```python
from build123d import *

# Parameters (mm, degrees)
BOSS_EXTRUDE1_DEPTH = 6.35
SKETCH2_R           = 1.27
CUT_EXTRUDE1_DEPTH  = 64.634002359


with BuildPart() as part:
    # Sketch1 → Boss-Extrude1 (new body)
    with BuildSketch(Plane.XY):
        with BuildLine():
            Line((52.3875, -33.02), (52.3875, 33.02))
            ThreePointArc((52.3875, 33.02), (51.643551224, 34.816051224), (49.8475, 35.56))
            Line((49.8475, 35.56), (-49.8475, 35.56))
            ThreePointArc((-49.8475, 35.56), (-51.643551224, 34.816051224), (-52.3875, 33.02))
            Line((-52.3875, 33.02), (-52.3875, -33.02))
            ThreePointArc((-52.3875, -33.02), (-51.643551224, -34.816051224), (-49.8475, -35.56))
            Line((-49.8475, -35.56), (49.8475, -35.56))
            ThreePointArc((49.8475, -35.56), (51.643551224, -34.816051224), (52.3875, -33.02))
        make_face()
        with BuildLine():
            Line((-38.502324621, 28.736218676), (13.971672014, 28.736218676))
            ThreePointArc((13.971672014, 28.736218676), (14.869697627, 28.364244288), (15.241672014, 27.466218676))
            Line((15.241672014, 27.466218676), (15.241672014, 21.89465856))
            ThreePointArc((15.241672014, 21.89465856), (14.869697627, 20.996632948), (13.971672014, 20.62465856))
            Line((13.971672014, 20.62465856), (-38.502324621, 20.62465856))
            ThreePointArc((-38.502324621, 20.62465856), (-39.400350233, 20.996632948), (-39.772324621, 21.89465856))
            Line((-39.772324621, 21.89465856), (-39.772324621, 27.466218676))
            ThreePointArc((-39.772324621, 27.466218676), (-39.400350233, 28.364244288), (-38.502324621, 28.736218676))
        make_face(mode=Mode.SUBTRACT)
        with BuildLine():
            Line((1.27, -9.646243467), (12.539518383, -9.646243467))
            ThreePointArc((12.539518383, -9.646243467), (13.437543995, -10.018217855), (13.809518383, -10.916243467))
            Line((13.809518383, -10.916243467), (13.809518383, -27.94))
            ThreePointArc((13.809518383, -27.94), (13.437543995, -28.838025612), (12.539518383, -29.21))
            Line((12.539518383, -29.21), (1.27, -29.21))
            ThreePointArc((1.27, -29.21), (0.371974388, -28.838025612), (0, -27.94))
            Line((0, -27.94), (0, -10.916243467))
            ThreePointArc((0, -10.916243467), (0.371974388, -10.018217855), (1.27, -9.646243467))
        make_face(mode=Mode.SUBTRACT)
    extrude(amount=BOSS_EXTRUDE1_DEPTH)

    # Sketch2 → Cut-Extrude1 (cut, through all)
    with BuildSketch(Plane.XY.offset(6.35)):
        with Locations((-49.3395, -22.86)):
            Circle(SKETCH2_R)
        with Locations((-49.3395, 22.86)):
            Circle(SKETCH2_R)
        with Locations((49.3395, 22.86)):
            Circle(SKETCH2_R)
        with Locations((49.3395, -22.86)):
            Circle(SKETCH2_R)
    extrude(amount=-CUT_EXTRUDE1_DEPTH, mode=Mode.SUBTRACT)


solid = part.part
```
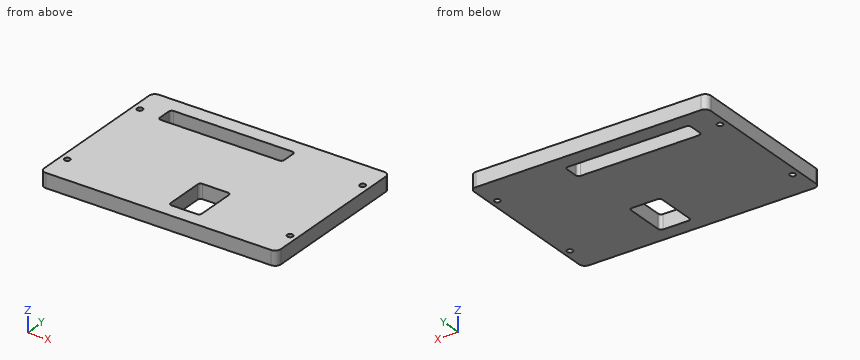
Geometry check sheet. Reference: the model listing, model coordinates, mm. Coordinates: 2 decimals unless noted, no trailing zeros. Order: outer loops, then holes, each group sorted by start corner. A loop starts at its lowest first (then second) coordinate and runs counter-clockwise, first axis right, second up. Notation, with made-up numbers: M 15.5,-10 L 34.5,-10 A17 ccw 34.5,-3 Z; hole C 75.5,-29.75 d2. An arc over 180 degrees is marked long. Answer as a JSON object with one key per item and string values.
Q1. Depth check by flat-ended pin: pin 1 Ø8 at (x, y) = (13.5, 22.5) entering from -Z. Enter the tip coordinate at first touch or a pass-through.
Results are:
{"pin 1": "stops at z = 0"}
Q2. Cross-section at A-A on y = -22.86. Record the cut outline in (x, z).
Results are:
{"outline": "M -52.39,0 L -50.61,0 L -50.61,6.35 L -52.39,6.35 Z; M -48.07,0 L 0,0 L 0,6.35 L -48.07,6.35 Z; M 13.81,0 L 48.07,0 L 48.07,6.35 L 13.81,6.35 Z; M 50.61,0 L 52.39,0 L 52.39,6.35 L 50.61,6.35 Z"}
Q3. Cross-section at B-B on z = 2. Record the cut outline in (x, y).
Results are:
{"outline": "M -52.39,-33.02 A2.54 ccw -49.85,-35.56 L 49.85,-35.56 A2.54 ccw 52.39,-33.02 L 52.39,33.02 A2.54 ccw 49.85,35.56 L -49.85,35.56 A2.54 ccw -52.39,33.02 Z; hole C -49.34,-22.86 d2.54; hole C -49.34,22.86 d2.54; hole M -39.77,21.89 A1.27 ccw -38.5,20.62 L 13.97,20.62 A1.27 ccw 15.24,21.89 L 15.24,27.47 A1.27 ccw 13.97,28.74 L -38.5,28.74 A1.27 ccw -39.77,27.47 Z; hole M 0,-27.94 A1.27 ccw 1.27,-29.21 L 12.54,-29.21 A1.27 ccw 13.81,-27.94 L 13.81,-10.92 A1.27 ccw 12.54,-9.65 L 1.27,-9.65 A1.27 ccw 0,-10.92 Z; hole C 49.34,-22.86 d2.54; hole C 49.34,22.86 d2.54"}
Q4. Scan lines: line 1 (Y direction, x = 10, z = 3.5); line 2 (Y direction, x = -10, z = 1); line 3 (X direction, y = -26, z = 1.5). Record each from-to range of solid material in increasing order.
Results are:
{"line 1": "y = -35.56 to -29.21, -9.65 to 20.62, 28.74 to 35.56", "line 2": "y = -35.56 to 20.62, 28.74 to 35.56", "line 3": "x = -52.39 to 0, 13.81 to 52.39"}
Q5. Cross-section at C-C on x = -17.5. Record the cut outline in (y, z).
Results are:
{"outline": "M -35.56,0 L 20.62,0 L 20.62,6.35 L -35.56,6.35 Z; M 28.74,0 L 35.56,0 L 35.56,6.35 L 28.74,6.35 Z"}
Q6. Cross-section at D-D on x = 10.5. Record the cut outline in (y, z), and give its area (3 significant figures).
Results are:
{"outline": "M -35.56,0 L -29.21,0 L -29.21,6.35 L -35.56,6.35 Z; M -9.65,0 L 20.62,0 L 20.62,6.35 L -9.65,6.35 Z; M 28.74,0 L 35.56,0 L 35.56,6.35 L 28.74,6.35 Z", "area": "276 mm²"}
